Here's how the part is built. I have some questions about the finished solid (model axes, mm). Coordinates: 2 decimals unless noted, no trailing zeros. Write each loop counter-clockwise with the first axis right and the second up, starting at its lowest first coordinate (ties: lowest second). Pieces come first, ordered by that corner, then holes.
(1) Imagine slicing it at D-D, the plane x = 0. List the corners of the cut face in (y, z) for me.
(2) Please list where these lines run through material, in increasing order: probe 1 along Y at (x, z) = (2.75, 1.1); probe 2 along Y at (x, z) = (-3.5, 0.5); probe 3 along X at (y, z) = (-0.8, 0.7).
(3) Imagine slicing it at B-B, the plane y = -1.5. List the corners of the cut face in (x, z) for me.
(4) Imagine slicing it at A-A, the plane x = 7.5. List the corners of the cut face in (y, z) for me, plus the area to 3 significant figures.
(5) Imagine slicing it at C-C, the plane z = 0.95. List the corners of the cut face in (x, y) for me (3 decimals).
```python
from build123d import *

# Parameters (mm, degrees)
SKETCH_1_R      = 1
EXTRUDE_1_DEPTH = 1.2


with BuildPart() as part:
    # Эскиз1 → Бобышка-Вытянуть1 (new body)
    with BuildSketch(Plane.XY):
        with BuildLine():
            Line((-1.5, -11.384990922), (-1.5, -10.585703858))
            ThreePointArc((-1.5, -10.585703858), (-1.710213715, -9.972321739), (-2.252475248, -9.616822288))
            ThreePointArc((-2.252475248, -9.616822288), (0, 8.3), (2.252475248, -9.616822288))
            ThreePointArc((2.252475248, -9.616822288), (1.710213715, -9.972321739), (1.5, -10.585703858))
            Line((1.5, -10.585703858), (1.5, -11.384990922))
            ThreePointArc((1.5, -11.384990922), (3.52665001, -13.346900966), (5.421753104, -11.257646183))
            ThreePointArc((5.421753104, -11.257646183), (5.685775429, -9.818447988), (6.599152829, -8.675320279))
            ThreePointArc((6.599152829, -8.675320279), (0, 10.9), (-6.599152829, -8.675320279))
            ThreePointArc((-6.599152829, -8.675320279), (-5.685775429, -9.818447988), (-5.421753104, -11.257646183))
            ThreePointArc((-5.421753104, -11.257646183), (-3.52665001, -13.346900966), (-1.5, -11.384990922))
        make_face()
        with Locations((-3.462944082, -11.384990922)):
            Circle(SKETCH_1_R, mode=Mode.SUBTRACT)
        with Locations((3.462944082, -11.384990922)):
            Circle(SKETCH_1_R, mode=Mode.SUBTRACT)
    extrude(amount=EXTRUDE_1_DEPTH)


solid = part.part
```
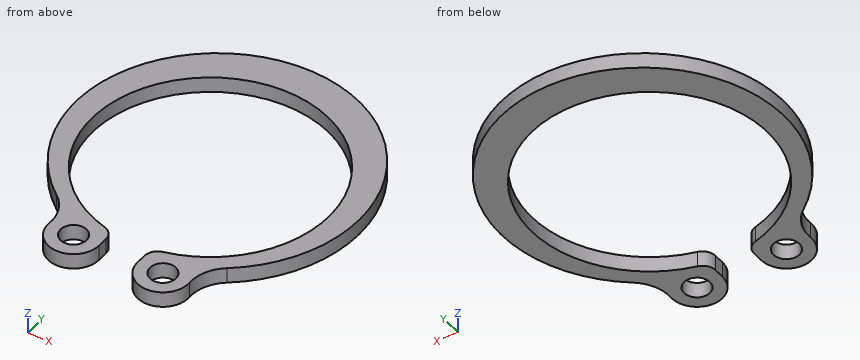
Recorded:
1. outline: (8.3, 0) - (10.9, 0) - (10.9, 1.2) - (8.3, 1.2) - close
2. probe 1: y = -13.21 to -12.09, -10.68 to -9.47, 7.87 to 10.55
2. probe 2: y = -13.35 to -12.38, -10.39 to -9.2, 7.6 to 10.32
2. probe 3: x = -10.87 to -9.1, 9.1 to 10.87
3. outline: (-10.8, 0) - (-9.07, 0) - (-9.07, 1.2) - (-10.8, 1.2) - close; (9.07, 0) - (10.8, 0) - (10.8, 1.2) - (9.07, 1.2) - close
4. outline: (-7.91, 0) - (-5.95, 0) - (-5.95, 1.2) - (-7.91, 1.2) - close; (4.35, 0) - (7.91, 0) - (7.91, 1.2) - (4.35, 1.2) - close
4. area: 6.61 mm2
5. outline: (-6.599, -8.675) arc R3 cw to (-5.422, -11.258) arc R1.963 ccw (long way) to (-1.5, -11.385) - (-1.5, -10.586) arc R1 ccw to (-2.252, -9.617) arc R9.1 cw (long way) to (2.252, -9.617) arc R1 ccw to (1.5, -10.586) - (1.5, -11.385) arc R1.963 ccw (long way) to (5.422, -11.258) arc R3 cw to (6.599, -8.675) arc R10.9 ccw (long way) to start; hole circle Ø2 at (-3.463, -11.385); hole circle Ø2 at (3.463, -11.385)
